Autodesk Inventor part; units mm, degrees
ref_plane "YZ Plane" through (0, 0, 0) normal (1, 0, 0) x (0, 1, 0)
ref_plane "XZ Plane" through (0, 0, 0) normal (0, 1, 0) x (-1, 0, 0)
ref_plane "XY Plane" through (0, 0, 0) normal (0, 0, 1) x (1, 0, 0)
sketch "Sketch2" plane through (0, 0, 0) normal (0, 1, 0) x (-1, 0, 0)
  line L0 (0, 0) -> (46, 0)
  line L1 (46, 0) -> (46, -46)
  line L2 (46, -46) -> (0, -46)
  line L3 (0, -46) -> (0, 0)
  dimension "d0" = 46
  dimension "d1" = 46
extrude "Extrusion1" add sketch "Sketch2" along normal blind 3.5
sketch "Sketch6" plane through (0, 0, 0) normal (0, -1, 0) x (1, 0, 0)
  line L0 (-13.25, -13.25) -> (-32.75, -13.25)
  line L1 (-32.75, -13.25) -> (-32.75, -32.75)
  line L2 (-32.75, -32.75) -> (-13.25, -32.75)
  line L3 (-13.25, -32.75) -> (-13.25, -13.25)
  line L4 (-46, -46) -> (0, -46)
  line L5 (0, 0) -> (0, -46)
  line L6 (-46, -46) -> (-46, 0)
  line L7 (0, 0) -> (-46, 0)
  line L8 (-46, 0) -> (-46, -46)
  line L9 (-46, -46) -> (0, -46)
  line L10 (0, -46) -> (0, 0)
  dimension "d41" = 13.25
  dimension "d42" = 13.25
  dimension "d43" = 13.25
  dimension "d44" = 13.25
extrude "Extrusion3" add sketch "Sketch6" along normal blind 1
sketch "Sketch7" plane through (0, -1, 0) normal (0, -1, 0) x (1, 0, 0)
  circle A0 centre (-6, -40) radius 3.25
  line L0 (-46, -46) -> (0, -46)
  line L1 (0, -46) -> (0, 0)
  circle A1 centre (-40, -40) radius 3.25
  line L2 (-46, 0) -> (-46, -46)
  circle A2 centre (-40, -6) radius 3.25
  line L3 (0, 0) -> (-46, 0)
  circle A3 centre (-6, -6) radius 3.25
  dimension "d26" = 6.5
  dimension "d27" = 6
  dimension "d28" = 6
  dimension "d29" = 6.5
  dimension "d30" = 6
  dimension "d31" = 6.5
  dimension "d32" = 6
  dimension "d33" = 6.5
  dimension "d45" = 6
  dimension "d46" = 6
  dimension "d47" = 6
  dimension "d48" = 6
hole "Hole2" at (-6, -1, -6) at (-6, -1, -40) at (-40, -1, -40) at (-40, -1, -6) direction (0, 1, 0) diameter 6.5 depth 9
sketch "Sketch8" plane through (0, 0, 0) normal (0, -1, 0) x (1, 0, 0)
  line L0 (-32.75, -13.25) -> (-13.25, -13.25)
  line L1 (-23, -13.25) -> (-23, -32.75)
  line L2 (-32.75, -32.75) -> (-13.25, -32.75)
  line L3 (-23, -23) -> (-11, -23)
  circle A0 centre (-17, -23) radius 2.125
  circle A1 centre (-23, -17) radius 2.125
  circle A2 centre (-23, -29) radius 2.125
  circle A3 centre (-29, -23) radius 2.125
  point P0 (0, 0)
  dimension "d49" = 4.25
  dimension "d50" = 6
  dimension "d51" = 4.25
  dimension "d52" = 6
  dimension "d53" = 4.25
  dimension "d54" = 6
  dimension "d55" = 4.25
  dimension "d56" = 6
hole "Hole3" at (-29, 0, -23) at (-23, 0, -17) at (-23, 0, -29) at (-17, 0, -23) direction (0, 1, 0) diameter 4.25 end through all
sketch "Sketch9" plane through (0, -1, 0) normal (0, -1, 0) x (1, 0, 0)
  line L0 (0, 0) -> (-46, 0)
  line L1 (0, 0) -> (-12.5, 0)
  line L2 (-12.5, 0) -> (-12.5, -12.5)
  line L3 (-12.5, -12.5) -> (0, -12.5)
  line L4 (0, -12.5) -> (0, 0)
  line L5 (-46, -46) -> (0, -46)
  line L6 (0, -46) -> (-12.5, -46)
  line L7 (-12.5, -46) -> (-12.5, -33.5)
  line L8 (-12.5, -33.5) -> (0, -33.5)
  line L9 (0, -33.5) -> (0, -46)
  line L10 (-46, -46) -> (-33.5, -46)
  line L11 (-33.5, -46) -> (-33.5, -33.5)
  line L12 (-33.5, -33.5) -> (-46, -33.5)
  line L13 (-46, -33.5) -> (-46, -46)
  circle A0 centre (-40, -40) radius 3.25
  circle A1 centre (-40, -40) radius 3.25
  circle A2 centre (-40, -6) radius 3.25
  circle A3 centre (-40, -6) radius 3.25
  circle A4 centre (-6.25, -40) radius 3.25
  circle A5 centre (-6.25, -6) radius 3.25
  line L14 (-46, 0) -> (-33.5, 0)
  line L15 (-33.5, 0) -> (-33.5, -12.5)
  line L16 (-33.5, -12.5) -> (-46, -12.5)
  line L17 (-46, -12.5) -> (-46, 0)
  dimension "d66" = 12.5
  dimension "d67" = 12.5
  dimension "d68" = 12.5
  dimension "d69" = 12.5
  dimension "d70" = 12.5
  dimension "d71" = 12.5
  dimension "d72" = 6.5
  dimension "d73" = 6.5
  dimension "d74" = 6.5
  dimension "d77" = 12.5
  dimension "d78" = 12.5
extrude "Extrusion4" add sketch "Sketch9" along normal blind 2.5
properties part number "RotatorBottom"
The model under review builds one solid part; all positions refer to its coordinate system, in mm. A direction names the side the tool comes from. Coordinates: 2 decimals unless noted, no trailing zeros. Write each loop counter-clockwise with the first axis right and the second up, starting at its lowest first coordinate (ties: lowest second). Pieces come first, ordered by that corner, then holes. Notation, with made-up numbers: (42, -1.5) - (93, -1.5) arc R10 ccw to (93, 3.5) - close; hole circle Ø10 at (-34, -31). An arc over 180 degrees is marked (long way). Answer as CSV lines item,"result".
(1) We need section A-A (y = -2.25). Give the boundary of the cut face in (x, z).
Data:
outline,"(-46, -46) - (-33.5, -46) - (-33.5, -33.5) - (-46, -33.5) - close; (-46, -12.5) - (-33.5, -12.5) - (-33.5, 0) - (-46, 0) - close; (-12.5, -46) - (0, -46) - (0, -33.5) - (-12.5, -33.5) - close; (-12.5, -12.5) - (0, -12.5) - (0, 0) - (-12.5, 0) - close; hole circle Ø6.5 at (-40, -40); hole circle Ø6.5 at (-40, -6); hole circle Ø6.5 at (-6.25, -40); hole circle Ø6.5 at (-6.25, -6)"
(2) Tool access review of faces 1 (the cylindrical face through (-17.093, 1.774, -20.877)), 2 (the flat face through (-12.5, -2, -40)), 3 (the flat face through (-40, -2, -33.5)), 4 (the flat face through (-38, -3.5, -9)), 5 (the flat face through (-13.25, -0.5, -23.1)): name each direction out of +Z, -Z, +X, -X, +Y, -Y from which nothing blocks a thin tool from reaching the whole face with its end or side.
Data:
face 1,"+Y, -Y"
face 2,"+Z, -Z, -Y"
face 3,"+X, -X, -Y"
face 4,"+Z, -Z, +X, -X, -Y"
face 5,"-Y"
(3) Clearance check with flat-ended pins moving along their axes: pin 1 Ø4 at (x, z) = (-36, -25.5) entering from -Y; pin 2 Ø4 at (x, z) = (-40, -6) entering from +Y; pin 3 Ø2 at (x, z) = (-19.5, -18) entering from -Y; pin 4 Ø1.7 at (x, z) = (-4, -7) entering from +Y. State where each tip first meets the part, or that it passes through.
Data:
pin 1,"stops at y = -1"
pin 2,"passes through"
pin 3,"stops at y = 0"
pin 4,"stops at y = -1"
(4) We need section B-B (x = -23). Give the boundary of the cut face in (y, z) (3 decimals).
Data:
outline,"(-1, -46) - (3.5, -46) - (3.5, -31.125) - (0, -31.125) - (0, -32.75) - (-1, -32.75) - close; (-1, -13.25) - (0, -13.25) - (0, -14.875) - (3.5, -14.875) - (3.5, 0) - (-1, 0) - close; (0, -26.875) - (3.5, -26.875) - (3.5, -19.125) - (0, -19.125) - close"
(5) We need section C-C (z = -17). Give the boundary of the cut face in (x, y) (3 decimals).
Data:
outline,"(-46, -1) - (-32.75, -1) - (-32.75, 0) - (-25.125, 0) - (-25.125, 3.5) - (-46, 3.5) - close; (-20.875, 0) - (-13.25, 0) - (-13.25, -1) - (0, -1) - (0, 3.5) - (-20.875, 3.5) - close"
(6) Mouldability with a two-part tool opening along Z and no side actions: class faces 6 (the flat face through (-46, 1, -23)), 7 (the cylindrical face through (-6.98, 1.28, -9.1)), 8 (the flat face through (-23, 1, -46)) as pulls with the +Z half, pulls with the -Z half, needs draft (parallel to the pull), parting line crosses it, or undercut.
Data:
face 6,"needs draft"
face 7,"undercut"
face 8,"pulls with the -Z half"
(7) We need section D-D (x = -17). Give the boundary of the cut face in (y, z) (3 decimals).
Data:
outline,"(-1, -46) - (3.5, -46) - (3.5, -25.125) - (0, -25.125) - (0, -32.75) - (-1, -32.75) - close; (-1, -13.25) - (0, -13.25) - (0, -20.875) - (3.5, -20.875) - (3.5, 0) - (-1, 0) - close"
(8) For line 1 along X through (y, z) = (-2.2, -40); line 2 along X through (y, z) = (1.5, -23) (3 decimals); line 3 along Z through (x, y) = (-6, 1.7), list the stretches that pass through material, from the lowest coordinate up. Write a range as [from, to].
Data:
line 1,"x = [-46, -43.25], [-36.75, -33.5], [-12.5, -9.5], [-3, 0]"
line 2,"x = [-46, -31.125], [-26.875, -19.125], [-14.875, 0]"
line 3,"z = [-46, -43.25], [-36.75, -9.25], [-2.75, 0]"
